Here's how the part is built. I have some questions about the finished solid (model axes, mm). Round coordinates to 2 decimals unless told otherwise and drop trailing zeros. Order: outer loops, then holes, each group sorted by start corner. A loop starts at its lowest first (then second) coordinate and runs counter-clockwise, first axis right, second up. Notation, with made-up numbers: (67.5, 72) -> (114.5, 72) arc R10 cw to (114.5, 77) -> close; hole circle Ø4 at (-40, 13.5). An arc over 180 degrees is marked (long way). Answer in a Markdown table with one row per item.
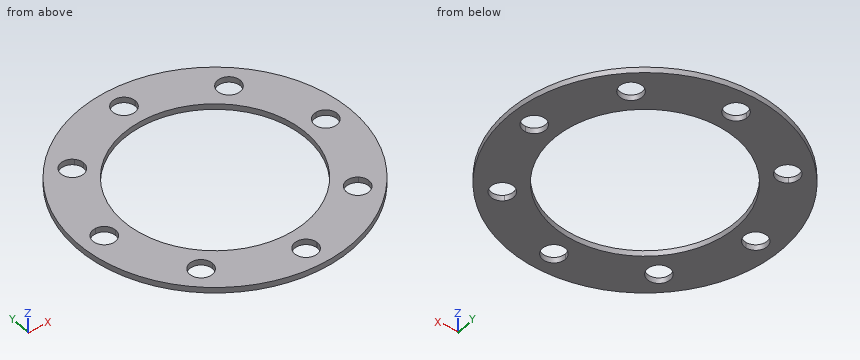
```python
from build123d import *

# Parameters (mm, degrees)
F0_R     = 120
F1_DEPTH = 5
F0_R_2   = 80
F2_DEPTH = 5


with BuildPart() as f1:
    # F0 (on Top) → F1 (new body)
    with BuildSketch(Plane.XY):
        Circle(F0_R)
        with BuildLine():
            ThreePointArc((76.146291, 64.820848), (91.609258, 40.096681), (99.281886, 11.962742))
            ThreePointArc((99.281886, 11.962742), (106.799943, 9.30097), (109.980254, 1.987158))
            ThreePointArc((109.980254, 1.987158), (106.943933, -5.189692), (99.67882, -8.008298))
            ThreePointArc((99.67882, -8.008298), (93.130163, -36.424892), (78.661831, -61.743959))
            ThreePointArc((78.661831, -61.743959), (81.201294, -65.144284), (82.101848, -69.291583))
            ThreePointArc((82.101848, -69.291583), (75.788988, -78.587012), (64.820848, -76.146291))
            ThreePointArc((64.820848, -76.146291), (40.096681, -91.609258), (11.962742, -99.281886))
            ThreePointArc((11.962742, -99.281886), (11.981052, -99.630856), (11.987158, -99.980254))
            ThreePointArc((11.987158, -99.980254), (1.836424, -109.979118), (-8.008298, -99.67882))
            ThreePointArc((-8.008298, -99.67882), (-36.424892, -93.130163), (-61.743959, -78.661831))
            ThreePointArc((-61.743959, -78.661831), (-76.220741, -79.312033), (-76.146291, -64.820848))
            ThreePointArc((-76.146291, -64.820848), (-91.609258, -40.096681), (-99.281886, -11.962742))
            ThreePointArc((-99.281886, -11.962742), (-109.978279, -2.185874), (-99.67882, 8.008298))
            ThreePointArc((-99.67882, 8.008298), (-93.130163, 36.424892), (-78.661831, 61.743959))
            ThreePointArc((-78.661831, 61.743959), (-79.312033, 76.220741), (-64.820848, 76.146291))
            ThreePointArc((-64.820848, 76.146291), (-40.096681, 91.609258), (-11.962742, 99.281886))
            ThreePointArc((-11.962742, 99.281886), (-2.336555, 109.974148), (8.012842, 99.980254))
            ThreePointArc((8.012842, 99.980254), (8.011706, 99.82952), (8.008298, 99.67882))
            ThreePointArc((8.008298, 99.67882), (36.424892, 93.130163), (61.743959, 78.661831))
            ThreePointArc((61.743959, 78.661831), (72.793279, 81.468711), (79.291583, 72.101848))
            ThreePointArc((79.291583, 72.101848), (78.471645, 68.136189), (76.146291, 64.820848))
        make_face(mode=Mode.SUBTRACT)
    extrude(amount=F1_DEPTH)

    # F0 (on Top) → F2 (join)
    with BuildSketch(Plane.XY):
        with BuildLine():
            ThreePointArc((99.67882, -8.008298), (89.982229, 1.788442), (99.281886, 11.962742))
            ThreePointArc((99.281886, 11.962742), (91.609258, 40.096681), (76.146291, 64.820848))
            ThreePointArc((76.146291, 64.820848), (62.362425, 64.891664), (61.743959, 78.661831))
            ThreePointArc((61.743959, 78.661831), (36.424892, 93.130163), (8.008298, 99.67882))
            ThreePointArc((8.008298, 99.67882), (-1.788442, 89.982229), (-11.962742, 99.281886))
            ThreePointArc((-11.962742, 99.281886), (-40.096681, 91.609258), (-64.820848, 76.146291))
            ThreePointArc((-64.820848, 76.146291), (-62.806419, 72.978722), (-62.101848, 69.291583))
            ThreePointArc((-62.101848, 69.291583), (-67.954549, 60.192137), (-78.661831, 61.743959))
            ThreePointArc((-78.661831, 61.743959), (-93.130163, 36.424892), (-99.67882, 8.008298))
            ThreePointArc((-99.67882, 8.008298), (-92.803404, 4.976522), (-89.980254, -1.987158))
            ThreePointArc((-89.980254, -1.987158), (-92.666442, -8.806847), (-99.281886, -11.962742))
            ThreePointArc((-99.281886, -11.962742), (-91.609258, -40.096681), (-76.146291, -64.820848))
            ThreePointArc((-76.146291, -64.820848), (-65.325923, -62.921786), (-59.291583, -72.101848))
            ThreePointArc((-59.291583, -72.101848), (-59.92472, -75.603545), (-61.743959, -78.661831))
            ThreePointArc((-61.743959, -78.661831), (-36.424892, -93.130163), (-8.008298, -99.67882))
            ThreePointArc((-8.008298, -99.67882), (1.788442, -89.982229), (11.962742, -99.281886))
            ThreePointArc((11.962742, -99.281886), (40.096681, -91.609258), (64.820848, -76.146291))
            ThreePointArc((64.820848, -76.146291), (64.891664, -62.362425), (78.661831, -61.743959))
            ThreePointArc((78.661831, -61.743959), (93.130163, -36.424892), (99.67882, -8.008298))
        make_face()
        Circle(F0_R_2, mode=Mode.SUBTRACT)
    extrude(amount=F2_DEPTH)


solid = f1.part
```
1. Suppose I cut it at C-C on x = 5. Write out the boundary of the cut face in (y, z).
Numbers:
| item | result |
|---|---|
| outline | (-119.9, 0) -> (-109.52, 0) -> (-109.52, 5) -> (-119.9, 5) -> close; (-90.44, 0) -> (-79.84, 0) -> (-79.84, 5) -> (-90.44, 5) -> close; (79.84, 0) -> (92.83, 0) -> (92.83, 5) -> (79.84, 5) -> close; (107.13, 0) -> (119.9, 0) -> (119.9, 5) -> (107.13, 5) -> close |
2. Please list where these lines run through material, in increasing order: line 1 along Y through (x, z) = (64, 4.1); line 2 along Y through (x, z) = (0, 2.3); line 3 along X through (y, z) = (64.5, 1.8).
Numbers:
| item | result |
|---|---|
| line 1 | y = -101.51 to -75.15, -63.43 to -48, 48 to 63.62, 80.59 to 101.51 |
| line 2 | y = -120 to -109.78, -90.18 to -80, 80 to 90.18, 109.78 to 120 |
| line 3 | x = -101.19 to -80.88, -63.32 to -47.33, 47.33 to 62.79, 75.79 to 101.19 |
3. Suppose I cut it at A-A on x = -24. Write out the boundary of the cut face in (y, z), then the cut area to 3 significant figures.
Numbers:
| item | result |
|---|---|
| outline | (-117.58, 0) -> (-76.32, 0) -> (-76.32, 5) -> (-117.58, 5) -> close; (76.32, 0) -> (117.58, 0) -> (117.58, 5) -> (76.32, 5) -> close |
| area | 413 mm2 |
4. Suppose I cut it at D-D on y = -32. Write out the boundary of the cut face in (x, z).
Numbers:
| item | result |
|---|---|
| outline | (-115.65, 0) -> (-73.32, 0) -> (-73.32, 5) -> (-115.65, 5) -> close; (73.32, 0) -> (115.65, 0) -> (115.65, 5) -> (73.32, 5) -> close |
5. For pin 1 Ø1.5 at (y, z) = (44.5, 3.5) entering from -X; pin 2 Ø1 at (y, z) = (88.5, 2.5) entering from +X; pin 3 Ø1 at (y, z) = (18, 1.5) entering from +X, each with a flat end and sliding along its axis, tell me the tip position at first contact or that it passes through.
Numbers:
| item | result |
|---|---|
| pin 1 | stops at x = -111.74 |
| pin 2 | stops at x = 81.58 |
| pin 3 | stops at x = 118.72 |
6. Suppose I cut it at B-B on z = 3.9. State how many separate pieces and enclosed holes the cut face has, then the cut area to 3 significant figures.
Numbers:
| item | result |
|---|---|
| separate pieces | 1 |
| enclosed holes | 9 |
| area | 22,600 mm2 |
